```python
from build123d import *

# Parameters (mm, degrees)
SKETCH1_W                       = 304.8
SKETCH1_H                       = 203.2
BOSS_EXTRUDE1_DEPTH             = 5
CLEARANCE_HOLES_FOR_LED_PANEL_D = 2.2
M3_CLEARANCE_HOLE1_D            = 3.2
F_1_4_CLEARANCE_HOLE1_D         = 6.5278
F_3_8_CLEARANCE_HOLE1_D         = 9.8044


with BuildPart() as part:
    # Sketch1 → Boss-Extrude1 (new body)
    with BuildSketch(Plane(origin=(0, 0, 0), x_dir=(1, 0, 0), z_dir=(0, 1, 0))):
        with Locations((152.4, -101.6)):
            Rectangle(SKETCH1_W, SKETCH1_H)
    extrude(amount=BOSS_EXTRUDE1_DEPTH)

    # clearance holes for led panel (through all)
    with Locations(Plane(origin=(0, 5, 0), x_dir=(1, 0, 0), z_dir=(0, 1, 0))):
        with Locations((80, -106.2), (130, -106.2), (130, -152.2), (80, -152.2), (80, -198.2), (130, -198.2)):
            Hole(CLEARANCE_HOLES_FOR_LED_PANEL_D / 2)

    # M3 Clearance Hole1 (through all)
    with Locations(Plane(origin=(0, 5, 0), x_dir=(1, 0, 0), z_dir=(0, 1, 0))):
        with Locations((59, -112.2), (151, -112.2), (151, -193.2), (59, -193.2)):
            Hole(M3_CLEARANCE_HOLE1_D / 2)

    # 1/4 Clearance Hole1 (through all)
    with Locations(Plane(origin=(0, 5, 0), x_dir=(1, 0, 0), z_dir=(0, 1, 0))):
        with Locations((15.875, -187.4139), (288.925, -187.4139)):
            Hole(F_1_4_CLEARANCE_HOLE1_D / 2)

    # 3/8 Clearance Hole1 (through all)
    with Locations(Plane(origin=(0, 5, 0), x_dir=(1, 0, 0), z_dir=(0, 1, 0))):
        with Locations((28.575, -15.9639), (276.225, -15.9639)):
            Hole(F_3_8_CLEARANCE_HOLE1_D / 2)


solid = part.part
```
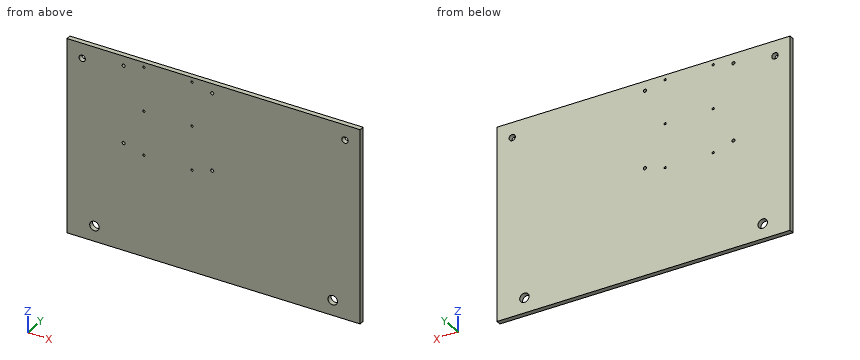
Geometry: final body of the model. Coordinates: model frame, mm. Give positions to 0.01 mm unless a question says otherwise; leave off trailing zeros. Write each loop counter-clockwise with the first axis right and the second up, starting at its lowest first coordinate (ties: lowest second). Pieces come first, ordered by that corner, then holes.
1. Line query: probe 1 along Z at (x, y) = (80, 2.1); probe 2 along X at (y, z) = (1.8, 187); probe 3 along X at (y, z) = (2.5, 152.2). Output: solid intervals per line, ascending.
2. Pin query (flat end, axial travel): P1, Ø1.3, axis at x = 80, z = 106.2, coming from the -Y side; P2, Ø3.5, axis at x = 80, z = 152.2, coming from the +Y side. Return the tip coordinate at first contact, or that it passes through.
3. Section query A-A, the plane x = 276.5. Return loops of the section in (y, z), then the cut area to 3 significant figures.
Computed:
1. probe 1: z = 0 to 105.1, 107.3 to 151.1, 153.3 to 197.1, 199.3 to 203.2
1. probe 2: x = 0 to 12.64, 19.11 to 285.69, 292.16 to 304.8
1. probe 3: x = 0 to 78.9, 81.1 to 128.9, 131.1 to 304.8
2. P1: passes through
2. P2: stops at y = 5
3. outline: (0, 0) - (5, 0) - (5, 11.07) - (0, 11.07) - close; (0, 20.86) - (5, 20.86) - (5, 203.2) - (0, 203.2) - close
3. area: 967 mm2
